Can you work these out from the model? Positions are in its coordinate system, mm. Give positions to 0.01 mm unless a question says otherwise; leave off trailing zeros. Write each loop counter-clockwise with the first axis right and the second up, starting at its lowest first coordinate (ties: lowest second). Pieces come first, ordered by that corner, then holes.
Autodesk Fusion 360 part; units mm, degrees
sketch "Sketch1" plane through (0, 0, 0) normal (0, 1, 0) x (1, 0, 0)
  circle A0 centre (0, 0) radius 5
  circle A1 centre (0, 0) radius 7.5
  dimension "d1" = 10
  dimension "d2" = 15
extrude "Extrude1" add sketch "Sketch1" along normal blind 14
sketch "Sketch2" plane through (0, 0, 0) normal (0, -1, 0) x (1, 0, 0)
  circle A0 centre (0, 0) radius 5
  circle A1 centre (0, 0) radius 7.5
  circle A2 centre (0, 0) radius 7.5
  circle A3 centre (0, 0) radius 12.5
  dimension "d5" = 25
chamfer "Chamfer1" distance 0.5 angle 45 2 edges at (-6.9925, 0, 2.7121) (-6.9925, 14, 2.7121)
extrude "Extrude2" add sketch "Sketch2" against normal blind 14 contours A3
chamfer "Chamfer2" distance 0.5 angle 45 4 edges at (-6.9925, 0, 2.7121) (-6.9925, 14, -2.7121) (-11.6541, 14, 4.5202) (-11.6541, 0, -4.5202)
sketch "Sketch3" plane through (0, 0, 0) normal (0, -1, 0) x (1, 0, 0)
  circle A0 centre (0, 0) radius 8
  circle A1 centre (0, 0) radius 12
  circle A2 centre (0, 0) radius 12.5
  circle A3 centre (0, 0) radius 15
  dimension "d10" = 25
  dimension "d11" = 30
extrude "Extrude3" add sketch "Sketch3" against normal blind 14 contours A3
chamfer "Chamfer3" distance 0.5 angle 45 2 edges at (-11.6541, 0, 4.5202) (-11.6541, 14, -4.5202)
chamfer "Chamfer4" distance 0.5 angle 45 4 edges at (-13.9849, 14, 5.4242) (-13.9849, 0, -5.4242) (-4.6616, 0, -1.8081) (-4.6616, 14, -1.8081)
1) For pin 1 Ø8 at (y, z) = (6.5, -0.5) entering from +X; pin 2 Ø1 at (x, y) = (-10, 9) entering from +Z; pin 3 Ø1.5 at (x, y) = (7.5, 6) entering from +Z; pin 4 Ø6 at (y, z) = (2, -10) entering from -X, each with a flat end and sliding along its axis, tell me the tip position at first contact or that it passes through.
Values follow:
pin 1: stops at x = 15
pin 2: stops at z = 11.61
pin 3: stops at z = 13.4
pin 4: stops at x = -13.27
2) If we mould it in two halves opening along X, with no side actions, what happens to faces 1 (the face through (-9, 14, 10)), 2 (the face through (-1.08, 6.91, -4.88)), 3 (the face through (-14.985, 6.909, 0.66))? For each: +X half, -X half, draft (parallel to the pull), parting line (faces both ways), or undercut.
Values follow:
face 1: draft
face 2: undercut
face 3: parting line
3) Please list where these lines run through material, in increasing order: L1, parallel to Z at x = 0, y = 4.75; L2, parallel to Z at x = -2.75, y = 1; L3, parallel to X at y = 4, z = -2.25.
Values follow:
L1: z = -15 to -5, 5 to 15
L2: z = -14.75 to -4.18, 4.18 to 14.75
L3: x = -14.83 to -4.47, 4.47 to 14.83
4) Suppose I cut it at A-A on y = 1.75. Write out the boundary of the cut face in (x, z), plus the area to 3 significant figures.
Values follow:
outline: circle Ø30 at (0, 0); hole circle Ø10 at (0, 0)
area: 628 mm2
